Work out the finished part from the listing and answer in its coordinate system (mm). Round coordinates to 2 decimals unless told otherwise and drop trailing zeros. Loops run counter-clockwise (first coordinate to the right, second up) from the corner with the lowest first, then second, coordinate; pieces in that order, holes last. Notation, with made-up numbers: (0, 74.5) - (58, 74.5) arc R12 ccw to (58, 81.5) - close; hole circle Ø6 at (65, 26.5). An arc over 180 degrees is marked (long way). Return JSON: item names as keys, results as strings.
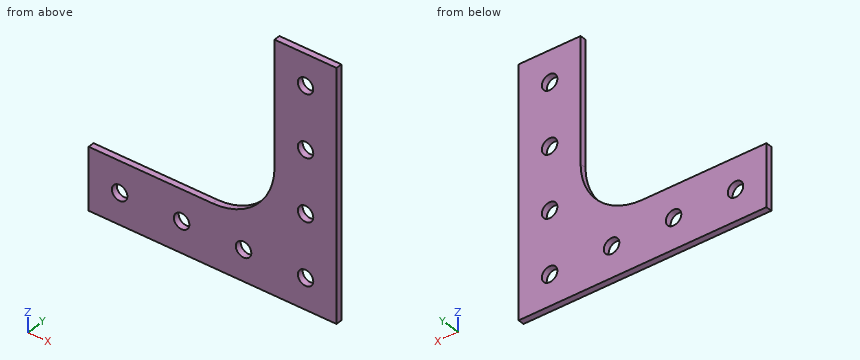
Autodesk Inventor part; units mm, degrees
ref_plane "YZ Plane" through (0, 0, 0) normal (1, 0, 0) x (0, 1, 0)
ref_plane "XZ Plane" through (0, 0, 0) normal (0, 1, 0) x (-1, 0, 0)
ref_plane "XY Plane" through (0, 0, 0) normal (0, 0, 1) x (1, 0, 0)
sketch "Sketch1" plane through (0, 0, 0) normal (0, 1, 0) x (-1, 0, 0)
  line L0 (0, 0) -> (0, 101.6)
  line L1 (0, 101.6) -> (25.4, 101.6)
  line L2 (0, 0) -> (101.6, 0)
  line L3 (101.6, 0) -> (101.6, 25.4)
  line L4 (50.8, 25.4) -> (101.6, 25.4)
  line L5 (25.4, 50.8) -> (25.4, 101.6)
  arc A0 (25.4, 28.575) -> (28.575, 25.4) centre (28.575, 28.575) ccw
  arc A1 (25.4, 50.8) -> (50.8, 25.4) centre (50.8, 50.8) ccw
  dimension "d0" = 101.6
  dimension "d1" = 25.4
  dimension "d2" = 101.6
  dimension "d3" = 25.4
  dimension "d4" = 3.175
  dimension "d5" = 25.4
extrude "Extrusion1" add sketch "Sketch1" along normal blind 2.54
hole "Hole1" at (-12.7, 2.54, 12.7) direction (0, -1, 0) diameter 6.35 end through all
pattern_linear "Rectangular Pattern1" count 4 spacing 25.4 along (-1, 0, 0) of "Hole1"
pattern_linear "Rectangular Pattern2" count 4 spacing 25.4 along (0, 0, 1) of "Hole1"
properties part number "Gusset"
1) Section C-C (y = 2.05) is taken. Give the vertices of the cut face in (x, z) (3 decimals), and give its area (3 significant figures).
Verdict:
{"outline": "(-101.6, 0) - (0, 0) - (0, 101.6) - (-25.4, 101.6) - (-25.4, 50.8) arc R25.4 cw to (-50.8, 25.4) - (-101.6, 25.4) - close; hole circle Ø6.35 at (-88.9, 12.7); hole circle Ø6.35 at (-63.5, 12.7); hole circle Ø6.35 at (-38.1, 12.7); hole circle Ø6.35 at (-12.7, 12.7); hole circle Ø6.35 at (-12.7, 38.1); hole circle Ø6.35 at (-12.7, 63.5); hole circle Ø6.35 at (-12.7, 88.9)", "area": "4,430 mm2"}
2) Section A-A (x = -88.9) is taken. Give the vertices of the cut face in (y, z) (3 decimals).
Verdict:
{"outline": "(0, 0) - (2.54, 0) - (2.54, 9.525) - (0, 9.525) - close; (0, 15.875) - (2.54, 15.875) - (2.54, 25.4) - (0, 25.4) - close"}
3) Find the intervals of material crossed by L1, parallel to X at y = 2, z = 12.7 (3 decimals); L2, parallel to Z at x = -12.7, y = 1.2 (3 decimals); L3, parallel to Z at x = -10.5, y = 0.3, in increasing order.
Verdict:
{"L1": "x = -101.6 to -92.075, -85.725 to -66.675, -60.325 to -41.275, -34.925 to -15.875, -9.525 to 0", "L2": "z = 0 to 9.525, 15.875 to 34.925, 41.275 to 60.325, 66.675 to 85.725, 92.075 to 101.6", "L3": "z = 0 to 10.41, 14.99 to 35.81, 40.39 to 61.21, 65.79 to 86.61, 91.19 to 101.6"}
4) Section B-B (z = 12.7) is taken. Give the vertices of the cut face in (x, y) (3 decimals).
Verdict:
{"outline": "(-101.6, 0) - (-92.075, 0) - (-92.075, 2.54) - (-101.6, 2.54) - close; (-85.725, 0) - (-66.675, 0) - (-66.675, 2.54) - (-85.725, 2.54) - close; (-60.325, 0) - (-41.275, 0) - (-41.275, 2.54) - (-60.325, 2.54) - close; (-34.925, 0) - (-15.875, 0) - (-15.875, 2.54) - (-34.925, 2.54) - close; (-9.525, 0) - (0, 0) - (0, 2.54) - (-9.525, 2.54) - close"}
5) Flat-ended cylindrical pins translate along their axes: pin 1 (1 mm diameter, centred on x = -44, y = 1.5, fed in from +Z); pin 2 (0.8 mm diameter, centred on y = 1, z = 67.5, fed in from -X). Find the tip coordinate at first contact, or state that the pin passes through.
Verdict:
{"pin 1": "stops at z = 26.47", "pin 2": "stops at x = -25.4"}
6) Section D-D (z = 88.9) is taken. Give the vertices of the cut face in (x, y) (3 decimals).
Verdict:
{"outline": "(-25.4, 0) - (-15.875, 0) - (-15.875, 2.54) - (-25.4, 2.54) - close; (-9.525, 0) - (0, 0) - (0, 2.54) - (-9.525, 2.54) - close"}
